Autodesk Inventor part; units mm, degrees
ref_plane "YZ Plane" through (0, 0, 0) normal (1, 0, 0) x (0, 1, 0)
ref_plane "XZ Plane" through (0, 0, 0) normal (0, 1, 0) x (-1, 0, 0)
ref_plane "XY Plane" through (0, 0, 0) normal (0, 0, 1) x (1, 0, 0)
sketch "Sketch1" plane through (0, 0, 0) normal (0, 1, 0) x (-1, 0, 0)
  line L0 (0, 0) -> (-30.48, 0)
  line L1 (-30.48, 0) -> (-30.48, -25.4)
  line L2 (-30.48, -25.4) -> (0, -25.4)
  line L3 (0, -25.4) -> (0, 0)
  line L4 (0, -25.4) -> (3.175, -25.4)
  line L5 (3.175, -25.4) -> (3.175, 0)
  line L6 (3.175, 0) -> (0, 0)
  line L7 (0, 0) -> (0, -25.4)
  line L8 (-30.48, -25.4) -> (-33.655, -25.4)
  line L9 (-33.655, -25.4) -> (-33.655, 0)
  line L10 (-33.655, 0) -> (-30.48, 0)
  line L11 (-30.48, 0) -> (-30.48, -25.4)
  dimension "d0" = 30.48
  dimension "d1" = 25.4
  dimension "d2" = 3.175
  dimension "d3" = 3.175
extrude "Extrusion1" add sketch "Sketch1" along normal blind 3.175 contours L3 L2 L1 L0
extrude "Extrusion2" add sketch "Sketch1" along normal blind 50.8 contours L6 L5 L4 L3 | L1 L8 L9 L10
sketch "Sketch2" plane through (-3.175, 0, -25.4) normal (-1, 0, 0) x (0, 0, 1)
  circle A0 centre (12.7, 38.1) radius 4.064
  line L0 (0, 50.8) -> (25.4, 50.8)
  line L1 (12.7, 38.1) -> (0, 38.1) construction
  line L2 (12.7, 38.1) -> (25.4, 38.1) construction
  point P0 (25.4, 0)
  dimension "d8" = 8.128
  dimension "d9" = 12.7
extrude "Extrusion3" cut sketch "Sketch2" against normal through all
fillet "Fillet1" radius 12.7 4 edges at (-1.5875, 50.8, 0) (32.0675, 50.8, 0) (32.0675, 50.8, -25.4) (-1.5875, 50.8, -25.4)
fillet "Fillet2" radius 6.35 4 edges at (-3.175, 0, -12.7) (0, 3.175, -12.7) (30.48, 3.175, -12.7) (33.655, 0, -12.7)
sketch "Sketch3" plane through (0, 0, 0) normal (0, -1, 0) x (1, 0, 0)
  circle A0 centre (14.605, -12.7) radius 2.921
  line L0 (14.605, -12.7) -> (1.905, -12.7) construction
  line L1 (27.305, 0) -> (27.305, -25.4) construction
  line L2 (3.175, 0) -> (27.305, 0) construction
  line L3 (3.175, -25.4) -> (3.175, 0) construction
  line L4 (27.305, -25.4) -> (3.175, -25.4) construction
  line L5 (14.605, -12.7) -> (27.305, -12.7) construction
  line L6 (14.605, -12.7) -> (14.605, 0) construction
  line L7 (14.605, -12.7) -> (14.605, -25.4) construction
  point P0 (0, 0)
  dimension "d14" = 5.842
extrude "Extrusion4" cut sketch "Sketch3" against normal through all
properties part number "MainMount" material "ABS Plastic"
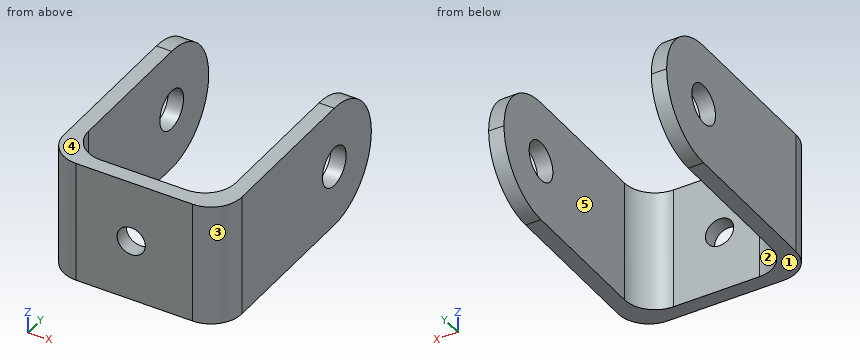
Input: part model. Units: mm. Frame: model coordinates. Face numbers are marked on the shaded views. A direction names the side the tool comes from. Coordinates: 2 decimals unless noted, no trailing zeros. Loops run counter-clockwise (first coordinate to the right, second up) from the corner with the lowest first, then second, coordinate; pieces in that order, holes last. Notation, with made-up numbers: (35.5, 16.25) -> (89.5, 16.25) arc R20 ccw to (89.5, 44.25) -> close; hole circle Ø1 at (72, 20). An arc over 180 degrees is marked (long way). Write each question's results on one line, items separated by ' | '. Start each with the question number.
Q1. Section A-A, the plane y = 29. Return the cut outline in (x, z) (3 decimals).
Q2. Ray query, line 1 (X direction, y = 43.5, z = -22.5) (3 decimals); line 2 (Y direction, x = 21, z = -15) (3 decimals); line 3 (Y direction, x = 31.35, z = -12.7). Return the intervals inside material, ascending. Write a range as from..to.
Q3. Reachability of the marked faces 4 and 5 from +Z, -Z, +X, -X, +Y, -Y: full face, straight path, thin tool, end or side. Return the list, or none.
Q4. Section C-C, the plane x = 23.5. Return the cut outline in (y, z) (3 decimals).
Q5. Pull-direction query (X, two-part tool) for the marked faces 1, 2 and 3; classes: released by +X, released by -X, zero draft, split by the parting line, or undercut.
Q6. Section B-B, the plane z = -19.75. Return the cut outline in (x, y) (3 decimals), plus the area to 3 significant figures.
Q7. Pin query (flat end, axial travel): pin 1 (1.5 mm diameter, centred on x = 16.5, z = -11.5, fed in from +Y) (3 decimals). Return the tip coordinate at first contact, or that it passes through.
Q8. Section D-D, the plane z = -2. Return the cut outline in (x, y) (3 decimals), plus the area to 3 significant figures.
Found:
1) outline: (-3.175, -25.4) -> (0, -25.4) -> (0, 0) -> (-3.175, 0) -> close; (30.48, -25.4) -> (33.655, -25.4) -> (33.655, 0) -> (30.48, 0) -> close
2) line 1: -3.175..0, 30.48..33.655 | line 2: 0..3.175 | line 3: 1.46..34.04, 42.16..50.8
3) face 4: +Z, +X, -X, +Y, -Y | face 5: +Z, -Z, +Y
4) outline: (0, -25.4) -> (3.175, -25.4) -> (3.175, 0) -> (0, 0) -> close
5) face 1: zero draft | face 2: undercut | face 3: released by +X
6) outline: (-3.175, 6.35) arc R6.35 ccw to (3.175, 0) -> (27.305, 0) arc R6.35 ccw to (33.655, 6.35) -> (33.655, 48.664) -> (30.48, 48.664) -> (30.48, 9.525) arc R6.35 cw to (24.13, 3.175) -> (6.35, 3.175) arc R6.35 cw to (0, 9.525) -> (0, 48.664) -> (-3.175, 48.664) -> close | area: 406 mm2
7) pin 1: y = 3.175
8) outline: (-3.175, 6.35) arc R6.35 ccw to (3.175, 0) -> (27.305, 0) arc R6.35 ccw to (33.655, 6.35) -> (33.655, 44.941) -> (30.48, 44.941) -> (30.48, 9.525) arc R6.35 cw to (24.13, 3.175) -> (6.35, 3.175) arc R6.35 cw to (0, 9.525) -> (0, 44.941) -> (-3.175, 44.941) -> close | area: 382 mm2
